The listing builds one solid part. Answer for the finished solid, in the listing's coordinates (mm). Face numbers are marked on the shaded views. A direction names the side the tool comes from. Coordinates: 2 decimals unless noted, no trailing zeros. Write each loop counter-clockwise with the first axis right and the second up, starting at its lowest first coordinate (ties: lowest second). Pieces come first, ordered by that corner, then holes.
from build123d import *

# Parameters (mm, degrees)
SKETCH1_W           = 20
SKETCH1_H           = 20
BOSS_EXTRUDE1_DEPTH = 10
SKETCH2_W           = 10
SKETCH2_H           = 10
BOSS_EXTRUDE2_DEPTH = 30
SKETCH3_W           = 5
SKETCH3_H           = 2
BOSS_EXTRUDE3_DEPTH = 3
SKETCH4_R           = 2.5
BOSS_EXTRUDE4_DEPTH = 2
SKETCH5_R           = 0.5
CUT_EXTRUDE1_DEPTH  = 10


with BuildPart() as part:
    # Sketch1 → Boss-Extrude1 (new body)
    with BuildSketch(Plane(origin=(0, 0, 0), x_dir=(1, 0, 0), z_dir=(0, 1, 0))):
        Rectangle(SKETCH1_W, SKETCH1_H)
    extrude(amount=BOSS_EXTRUDE1_DEPTH)

    # Sketch2 → Boss-Extrude2 (add)
    with BuildSketch(Plane(origin=(0, 10, 0), x_dir=(-1, 0, 0), z_dir=(0, -1, 0))):
        Rectangle(SKETCH2_W, SKETCH2_H)
    extrude(amount=-BOSS_EXTRUDE2_DEPTH)

    # Sketch3 → Boss-Extrude3 (add)
    with BuildSketch(Plane(origin=(0, 40, 0), x_dir=(1, 0, 0), z_dir=(0, 1, 0))):
        with Locations((0, 4)):
            Rectangle(SKETCH3_W, SKETCH3_H)
        with Locations((0, -4)):
            Rectangle(SKETCH3_W, SKETCH3_H)
    extrude(amount=BOSS_EXTRUDE3_DEPTH)

    # Sketch4 → Boss-Extrude4 (add)
    with BuildSketch(Plane(origin=(0, 0, -5), x_dir=(1, 0, 0), z_dir=(0, 0, -1))):
        with Locations((0, -43)):
            Circle(SKETCH4_R)
    boss_extrude4 = extrude(amount=-BOSS_EXTRUDE4_DEPTH)

    # Mirror1: Boss-Extrude4 across plane
    add(boss_extrude4.mirror(Plane.XY))

    # Sketch5 → Cut-Extrude1 (cut)
    with BuildSketch(Plane(origin=(0, 0, -5), x_dir=(-1, 0, 0), z_dir=(0, 0, -1))):
        with Locations((0, 43.589170062)):
            Circle(SKETCH5_R)
    extrude(amount=-CUT_EXTRUDE1_DEPTH, mode=Mode.SUBTRACT)


solid = part.part
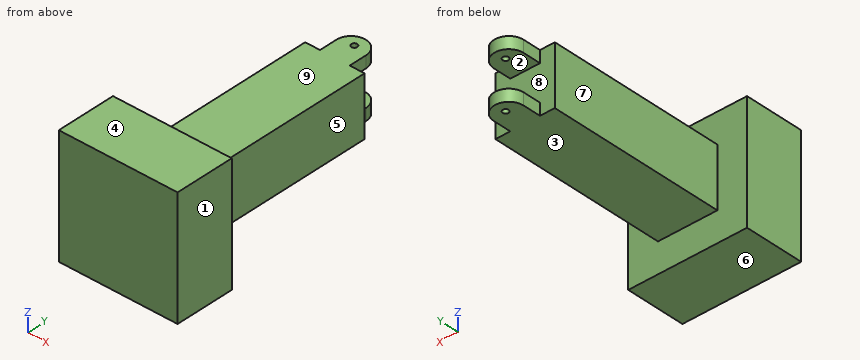
1. Section B-B on z = 4 is taken. Give the vertices of the cut face in (x, y).
Results found:
outline: (-10, 0) - (10, 0) - (10, 10) - (5, 10) - (5, 40) - (2.5, 40) - (2.5, 43) arc R2.5 ccw to (-2.5, 43) - (-2.5, 40) - (-5, 40) - (-5, 10) - (-10, 10) - close; hole circle Ø1 at (0, 43.59)
2. Section D-D on y = 39 is taken. Give the vertices of the cut face in (x, z).
Results found:
outline: (-5, -5) - (5, -5) - (5, 5) - (-5, 5) - close
3. Section A-A on x = 0 is taken. Give the vertices of the cut face in (y, z), then the cut area to 3 significant figures.
Results found:
outline: (0, -10) - (10, -10) - (10, -5) - (43.09, -5) - (43.09, -3) - (40, -3) - (40, 3) - (43.09, 3) - (43.09, 5) - (10, 5) - (10, 10) - (0, 10) - close; (44.09, -5) - (45.5, -5) - (45.5, -3) - (44.09, -3) - close; (44.09, 3) - (45.5, 3) - (45.5, 5) - (44.09, 5) - close
area: 518 mm2
4. For a pull along Z with two mould halves and no side action, classify the marked faces 6, 7, 8 and 9 as pulls with the +Z half, pulls with the -Z half, needs draft (parallel to the pull), parting line crosses it, or undercut.
Results found:
face 6: pulls with the -Z half
face 7: needs draft
face 8: undercut
face 9: pulls with the +Z half
5. Find the intervals of material crossed by L1, parallel to Y at x = 0, z = -3.4; L2, parallel to Y at x = 4.75, z = -6; L3, parallel to X at y = 29.5, z = 3, in increasing order.
Results found:
L1: y = 0 to 43.09, 44.09 to 45.5
L2: y = 0 to 10
L3: x = -5 to 5
6. Flat-ended cylindrical pins translate along their axes: P1, Ø3, axis at y = 23, z = 2, coming from the -X side; P2, Ø1.6, axis at y = 41, z = 4, coming from the +X side; P3, Ø2.5, axis at x = -1, y = 43, coming from the +Z side. Find the tip coordinate at first contact, or state that the pin passes through.
Results found:
P1: stops at x = -5
P2: stops at x = 2.5
P3: stops at z = 5
7. A tool of negligible diameter and unlimited length cuts with its end or side. For the marked faces 1, 2, 3, 4 and 5, from which of +Z, -Z, +X, -X, +Y, -Y can it reach the whole face along a straight path? Write none if from no direction.
Results found:
face 1: +Z, -Z, +X, +Y, -Y
face 2: +X, -X, +Y
face 3: -Z, +X, -X, +Y
face 4: +Z, +X, -X, +Y, -Y
face 5: +Z, -Z, +X, +Y
8. Section C-C on x = -4 is taken. Give the vertices of the cut face in (y, z), then the cut area to 3 significant figures.
Results found:
outline: (0, -10) - (10, -10) - (10, -5) - (40, -5) - (40, 5) - (10, 5) - (10, 10) - (0, 10) - close
area: 500 mm2
